Can you work these out from the model? Positions are in its coordinate system, mm. A direction names the side the tool comes from. Coordinates: 2 decimals unless noted, no trailing zeros. Write each loop counter-clockwise with the first axis right and the second up, starting at its lowest first coordinate (ties: lowest second). Pieces come first, ordered by that corner, then holes. Notation, with made-up numbers: (38.5, -39.75) -> (62.5, -39.75) arc R9 cw to (62.5, -30.75) -> close; hole circle Ø6 at (88.5, -20.5). An arc over 180 degrees is marked (long way). Use one line per item in the form item = value.
```python
from build123d import *

# Parameters (mm, degrees)
SKETCH1_R            = 1.5
SKETCH1_R_2          = 73
BOSS_EXTRUDE1_DEPTH  = 20
SKETCH7_R            = 73
SKETCH7_R_2          = 52.25
BOSS_EXTRUDE2_DEPTH  = 10
SKETCH8_R            = 73
BOSS_EXTRUDE3_DEPTH  = 10
BOSS_EXTRUDE4_DEPTH  = 20
SKETCH10_R           = 55.2
SKETCH10_R_2         = 52.25
CUT_EXTRUDE1_DEPTH   = 10
SKETCH11_R           = 40
CUT_EXTRUDE2_DEPTH   = 50
SKETCH12_R           = 3
SKETCH12_R_2         = 1.5
CUT_EXTRUDE3_DEPTH   = 3
SKETCH13_W           = 50
SKETCH13_H           = 6.823606938
BOSS_EXTRUDE5_DEPTH  = 5
BOSS_EXTRUDE6_DEPTH  = 5
BOSS_EXTRUDE7_DEPTH  = 5
BOSS_EXTRUDE8_DEPTH  = 5
SKETCH19_R           = 1.5
CUT_EXTRUDE4_DEPTH   = 5
SKETCH20_R           = 1.5
CUT_EXTRUDE5_DEPTH   = 5
SKETCH21_R           = 1.5
CUT_EXTRUDE6_DEPTH   = 5
SKETCH22_R           = 1.5
CUT_EXTRUDE7_DEPTH   = 5
SKETCH23_R           = 1.5
SKETCH23_R_2         = 1
BOSS_EXTRUDE9_DEPTH  = 5
SKETCH24_R           = 1.5
SKETCH24_R_2         = 1
BOSS_EXTRUDE10_DEPTH = 5
SKETCH25_R           = 1.5
SKETCH25_R_2         = 1
BOSS_EXTRUDE11_DEPTH = 5
SKETCH26_R           = 1.5
SKETCH26_R_2         = 1
BOSS_EXTRUDE12_DEPTH = 5


with BuildPart() as part:
    # Sketch1 → Boss-Extrude1 (new body)
    with BuildSketch(Plane(origin=(0, 0, 0), x_dir=(1, 0, 0), z_dir=(0, 1, 0))):
        with BuildLine():
            Line((77.460838348, -75.098177713), (77.460838348, 74.577424045))
            ThreePointArc((77.460838348, 74.577424045), (76.578174547, 76.708362964), (74.447235628, 77.591026765))
            Line((74.447235628, 77.591026765), (-75.22836613, 77.591026765))
            ThreePointArc((-75.22836613, 77.591026765), (-77.359305049, 76.708362964), (-78.24196885, 74.577424045))
            Line((-78.24196885, 74.577424045), (-78.24196885, -75.098177713))
            ThreePointArc((-78.24196885, -75.098177713), (-77.359305049, -77.229116632), (-75.22836613, -78.111780433))
            Line((-75.22836613, -78.111780433), (74.447235628, -78.111780433))
            ThreePointArc((74.447235628, -78.111780433), (76.578174547, -77.229116632), (77.460838348, -75.098177713))
        make_face()
        with Locations((-60.604326536, -60.47413812)):
            Circle(SKETCH1_R, mode=Mode.SUBTRACT)
        with Locations((-60.604326536, 59.953384452)):
            Circle(SKETCH1_R, mode=Mode.SUBTRACT)
        with Locations((59.823196035, 59.953384452)):
            Circle(SKETCH1_R, mode=Mode.SUBTRACT)
        with Locations((59.823196035, -60.47413812)):
            Circle(SKETCH1_R, mode=Mode.SUBTRACT)
        with Locations((-0.390565251, -0.260376834)):
            Circle(SKETCH1_R_2, mode=Mode.SUBTRACT)
    extrude(amount=BOSS_EXTRUDE1_DEPTH)

    # Sketch7 → Boss-Extrude2 (add)
    with BuildSketch(Plane(origin=(0, 20, 0), x_dir=(1, 0, 0), z_dir=(0, 1, 0))):
        with Locations((-0.390565251, -0.260376834)):
            Circle(SKETCH7_R)
        with Locations((-0.390565251, -0.260376834)):
            Circle(SKETCH7_R_2, mode=Mode.SUBTRACT)
    extrude(amount=-BOSS_EXTRUDE2_DEPTH)

    # Sketch8 → Boss-Extrude3 (add)
    with BuildSketch(Plane.XZ.offset(-10)):
        with Locations((-0.390565251, 0.260376834)):
            Circle(SKETCH8_R)
    extrude(amount=BOSS_EXTRUDE3_DEPTH)

    # Sketch9 → Boss-Extrude4 (add)
    with BuildSketch(Plane(origin=(0, 20, 0), x_dir=(1, 0, 0), z_dir=(0, 1, 0))):
        with BuildLine():
            ThreePointArc((-75.22836613, -78.111780433), (-77.359305049, -77.229116632), (-78.24196885, -75.098177713))
            Line((-78.24196885, -75.098177713), (-78.24196885, -78.111780433))
            Line((-78.24196885, -78.111780433), (-75.22836613, -78.111780433))
        make_face()
        with BuildLine():
            Line((77.460838348, -78.111780433), (77.460838348, -75.098177713))
            ThreePointArc((77.460838348, -75.098177713), (76.578174547, -77.229116632), (74.447235628, -78.111780433))
            Line((74.447235628, -78.111780433), (77.460838348, -78.111780433))
        make_face()
        with BuildLine():
            Line((77.460838348, 77.591026765), (74.447235628, 77.591026765))
            ThreePointArc((74.447235628, 77.591026765), (76.578174547, 76.708362964), (77.460838348, 74.577424045))
            Line((77.460838348, 74.577424045), (77.460838348, 77.591026765))
        make_face()
        with BuildLine():
            Line((-75.22836613, 77.591026765), (-78.24196885, 77.591026765))
            Line((-78.24196885, 77.591026765), (-78.24196885, 74.577424045))
            ThreePointArc((-78.24196885, 74.577424045), (-77.359305049, 76.708362964), (-75.22836613, 77.591026765))
        make_face()
    extrude(amount=-BOSS_EXTRUDE4_DEPTH)

    # Sketch10 → Cut-Extrude1 (cut)
    with BuildSketch(Plane(origin=(0, 20, 0), x_dir=(1, 0, 0), z_dir=(0, 1, 0))):
        with Locations((-0.390565251, -0.260376834)):
            Circle(SKETCH10_R)
        with Locations((-0.390565251, -0.260376834)):
            Circle(SKETCH10_R_2, mode=Mode.SUBTRACT)
    extrude(amount=-CUT_EXTRUDE1_DEPTH, mode=Mode.SUBTRACT)

    # Sketch11 → Cut-Extrude2 (cut)
    with BuildSketch(Plane(origin=(0, 20, 0), x_dir=(1, 0, 0), z_dir=(0, 1, 0))):
        with Locations((-0.390565251, -0.260376834)):
            Circle(SKETCH11_R)
    extrude(amount=-CUT_EXTRUDE2_DEPTH, mode=Mode.SUBTRACT)

    # Sketch12 → Cut-Extrude3 (cut)
    with BuildSketch(Plane(origin=(0, 20, 0), x_dir=(1, 0, 0), z_dir=(0, 1, 0))):
        with Locations((59.823196035, 59.953384452)):
            Circle(SKETCH12_R)
        with Locations((59.823196035, 59.953384452)):
            Circle(SKETCH12_R_2, mode=Mode.SUBTRACT)
        with Locations((-60.604326536, 59.953384452)):
            Circle(SKETCH12_R)
        with Locations((-60.604326536, 59.953384452)):
            Circle(SKETCH12_R_2, mode=Mode.SUBTRACT)
        with Locations((-60.604326536, -60.47413812)):
            Circle(SKETCH12_R)
        with Locations((-60.604326536, -60.47413812)):
            Circle(SKETCH12_R_2, mode=Mode.SUBTRACT)
        with Locations((59.823196035, -60.47413812)):
            Circle(SKETCH12_R)
        with Locations((59.823196035, -60.47413812)):
            Circle(SKETCH12_R_2, mode=Mode.SUBTRACT)
    extrude(amount=-CUT_EXTRUDE3_DEPTH, mode=Mode.SUBTRACT)

    # Sketch13 → Boss-Extrude5 (add)
    with BuildSketch(Plane.ZY.offset(78.24196885)):
        with Locations((0.260376834, 23.411803469)):
            Rectangle(SKETCH13_W, SKETCH13_H)
        Polygon((12.760376834, 32.49492606), (25.260376834, 26.823606938), (-24.739623166, 26.823606938), (-12.239623166, 32.49492606), align=None)
    extrude(amount=-BOSS_EXTRUDE5_DEPTH)

    # Sketch14 → Boss-Extrude6 (add)
    with BuildSketch(Plane(origin=(77.460838348, 0, 0), x_dir=(0, 0, -1), z_dir=(1, 0, 0))):
        Polygon((-25.260376834, 26.823606938), (-25.260376834, 20), (24.739623166, 20), (24.739623166, 26.823606938), (12.239623166, 32.49492606), (-12.760376834, 32.49492606), align=None)
    extrude(amount=-BOSS_EXTRUDE6_DEPTH)

    # Sketch17 → Boss-Extrude7 (add)
    with BuildSketch(Plane(origin=(0, 0, -77.591026765), x_dir=(-1, 0, 0), z_dir=(0, 0, -1))):
        Polygon((-77.460838348, 0), (78.24196885, 0), (78.24196885, 20), (25.390565251, 20), (25.390565251, 26.823606938), (12.890565251, 32.49492606), (-12.109434749, 32.49492606), (-24.609434749, 26.823606938), (-24.609434749, 20), (-77.460838348, 20), align=None)
    extrude(amount=-BOSS_EXTRUDE7_DEPTH)

    # Sketch18 → Boss-Extrude8 (add)
    with BuildSketch(Plane.XY.offset(78.111780433)):
        Polygon((-25.390565251, 20), (24.609434749, 20), (24.609434749, 26.823606938), (12.109434749, 32.49492606), (-12.890565251, 32.49492606), (-25.390565251, 26.823606938), align=None)
    extrude(amount=-BOSS_EXTRUDE8_DEPTH)

    # Sketch19 → Cut-Extrude4 (cut)
    with BuildSketch(Plane.ZY.offset(78.24196885)):
        with Locations((0.260376834, 26.24746303)):
            Circle(SKETCH19_R)
        with Locations((60.47413812, 10)):
            Circle(SKETCH19_R)
        with Locations((-59.953384452, 10)):
            Circle(SKETCH19_R)
    extrude(amount=-CUT_EXTRUDE4_DEPTH, mode=Mode.SUBTRACT)

    # Sketch20 → Cut-Extrude5 (cut)
    with BuildSketch(Plane(origin=(77.460838348, 0, 0), x_dir=(0, 0, -1), z_dir=(1, 0, 0))):
        with Locations((-60.47413812, 10)):
            Circle(SKETCH20_R)
        with Locations((59.953384452, 10)):
            Circle(SKETCH20_R)
        with Locations((-0.260376834, 26.24746303)):
            Circle(SKETCH20_R)
    extrude(amount=-CUT_EXTRUDE5_DEPTH, mode=Mode.SUBTRACT)

    # Sketch21 → Cut-Extrude6 (cut)
    with BuildSketch(Plane(origin=(0, 0, -77.591026765), x_dir=(-1, 0, 0), z_dir=(0, 0, -1))):
        with Locations((-59.823196035, 10)):
            Circle(SKETCH21_R)
        with Locations((0.390565251, 26.24746303)):
            Circle(SKETCH21_R)
        with Locations((60.604326536, 10)):
            Circle(SKETCH21_R)
    extrude(amount=-CUT_EXTRUDE6_DEPTH, mode=Mode.SUBTRACT)

    # Sketch22 → Cut-Extrude7 (cut)
    with BuildSketch(Plane.XY.offset(78.111780433)):
        with Locations((59.823196035, 10)):
            Circle(SKETCH22_R)
        with Locations((-0.390565251, 26.24746303)):
            Circle(SKETCH22_R)
        with Locations((-60.604326536, 10)):
            Circle(SKETCH22_R)
    extrude(amount=-CUT_EXTRUDE7_DEPTH, mode=Mode.SUBTRACT)

    # Sketch23 → Boss-Extrude9 (add)
    with BuildSketch(Plane.ZY.offset(78.24196885)):
        with Locations((60.47413812, 10)):
            Circle(SKETCH23_R)
        with Locations((60.47413812, 10)):
            Circle(SKETCH23_R_2, mode=Mode.SUBTRACT)
        with Locations((-59.953384452, 10)):
            Circle(SKETCH23_R)
        with Locations((-59.953384452, 10)):
            Circle(SKETCH23_R_2, mode=Mode.SUBTRACT)
        with Locations((0.260376834, 26.24746303)):
            Circle(SKETCH23_R)
        with Locations((0.260376834, 26.24746303)):
            Circle(SKETCH23_R_2, mode=Mode.SUBTRACT)
    extrude(amount=-BOSS_EXTRUDE9_DEPTH)

    # Sketch24 → Boss-Extrude10 (add)
    with BuildSketch(Plane.XY.offset(78.111780433)):
        with Locations((-60.604326536, 10)):
            Circle(SKETCH24_R)
        with Locations((-60.604326536, 10)):
            Circle(SKETCH24_R_2, mode=Mode.SUBTRACT)
        with Locations((-0.390565251, 26.24746303)):
            Circle(SKETCH24_R)
        with Locations((-0.390565251, 26.24746303)):
            Circle(SKETCH24_R_2, mode=Mode.SUBTRACT)
        with Locations((59.823196035, 10)):
            Circle(SKETCH24_R)
        with Locations((59.823196035, 10)):
            Circle(SKETCH24_R_2, mode=Mode.SUBTRACT)
    extrude(amount=-BOSS_EXTRUDE10_DEPTH)

    # Sketch25 → Boss-Extrude11 (add)
    with BuildSketch(Plane(origin=(77.460838348, 0, 0), x_dir=(0, 0, -1), z_dir=(1, 0, 0))):
        with Locations((-60.47413812, 10)):
            Circle(SKETCH25_R)
        with Locations((-60.47413812, 10)):
            Circle(SKETCH25_R_2, mode=Mode.SUBTRACT)
        with Locations((59.953384452, 10)):
            Circle(SKETCH25_R)
        with Locations((59.953384452, 10)):
            Circle(SKETCH25_R_2, mode=Mode.SUBTRACT)
        with Locations((-0.260376834, 26.24746303)):
            Circle(SKETCH25_R)
        with Locations((-0.260376834, 26.24746303)):
            Circle(SKETCH25_R_2, mode=Mode.SUBTRACT)
    extrude(amount=-BOSS_EXTRUDE11_DEPTH)

    # Sketch26 → Boss-Extrude12 (add)
    with BuildSketch(Plane(origin=(0, 0, -77.591026765), x_dir=(-1, 0, 0), z_dir=(0, 0, -1))):
        with Locations((-59.823196035, 10)):
            Circle(SKETCH26_R)
        with Locations((-59.823196035, 10)):
            Circle(SKETCH26_R_2, mode=Mode.SUBTRACT)
        with Locations((60.604326536, 10)):
            Circle(SKETCH26_R)
        with Locations((60.604326536, 10)):
            Circle(SKETCH26_R_2, mode=Mode.SUBTRACT)
        with Locations((0.390565251, 26.24746303)):
            Circle(SKETCH26_R)
        with Locations((0.390565251, 26.24746303)):
            Circle(SKETCH26_R_2, mode=Mode.SUBTRACT)
    extrude(amount=-BOSS_EXTRUDE12_DEPTH)


solid = part.part
```
Q1. If I drill on line 1 (Z direction, x = -59.5, y = 9); line 2 (Y direction, x = -41, z = 18.5); line 3 (X direction, y = 11, z = -23), over which ranges is the centre line in solid material (lowest first)? Write a range as from..to.
Return value:
line_1 = -77.59..-60.97, -58.94..59.46, 61.49..78.11
line_2 = 0..10
line_3 = -78.24..-50.45, 49.67..77.46
Q2. Suppose I cut it at C-C (y = 29.5). Write out the boundary of the cut face in (x, z), then the cut area to 3 significant figures.
Return value:
outline = (-78.24, -18.84) -> (-73.24, -18.84) -> (-73.24, 19.36) -> (-78.24, 19.36) -> close; (-19.49, -77.59) -> (18.71, -77.59) -> (18.71, -72.59) -> (-19.49, -72.59) -> close; (-19.49, 73.11) -> (18.71, 73.11) -> (18.71, 78.11) -> (-19.49, 78.11) -> close; (72.46, -18.84) -> (77.46, -18.84) -> (77.46, 19.36) -> (72.46, 19.36) -> close
area = 764 mm2
Q3. Thinking about a two-plate mould opening in X: for faces 1 (the flat face through (18.45, 29.62, 75.65)), 2 (the flat face through (75, 29.62, -18.58)), 3 (the flat face through (58, 17, 61)), which applies, released by +X, released by -X, zero draft, split by the parting line, or undercut?
Return value:
face_1 = released by +X
face_2 = zero draft
face_3 = undercut
Q4. For faces 4 (the flat face through (-25.391, 23, 76)), 5 (the flat face through (36.2, 10, -16.4)), 6 (the flat face through (-1, 25, 73.112)), which set-ups out of +Z, -Z, +X, -X, +Y, -Y let a thin tool reach every point of the face, with its end or its side?
Return value:
face_4 = +Z, -Z, -X, +Y
face_5 = +Y
face_6 = +X, -X, +Y
Q5. Suppose I cut it at A-A (x = 15). Write out the boundary of the cut face in (y, z), then the cut area to 3 significant figures.
Return value:
outline = (0, -77.59) -> (31.18, -77.59) -> (31.18, -72.59) -> (20, -72.59) -> (20, -52.75) -> (10, -52.75) -> (10, -36.66) -> (0, -36.66) -> close; (0, 37.18) -> (10, 37.18) -> (10, 53.27) -> (20, 53.27) -> (20, 73.11) -> (31.18, 73.11) -> (31.18, 78.11) -> (0, 78.11) -> close
area = 1,430 mm2
Q6. Will these pins go through, and if not, where does the flat tip stop? pin 1 (4 mm diameter, centred on x = 74.5, y = 23, fed in from -Z); pin 2 (1.8 mm diameter, centred on x = 60, z = 60.5, fed in from +Y); pin 3 (4 mm diameter, centred on x = -60.6, z = -59.95, fed in from +Y); pin 4 (1.6 mm diameter, centred on y = 10, z = -59.95, fed in from -X).
Return value:
pin_1 = -24.74
pin_2 = through
pin_3 = 17
pin_4 = -73.24
Q7. Suppose I cut it at D-D (y = 5). Write out the boundary of the cut face in (x, z), then the cut area to 3 significant figures.
Return value:
outline = (-78.24, -77.59) -> (77.46, -77.59) -> (77.46, 78.11) -> (-78.24, 78.11) -> close; hole circle Ø3 at (-60.6, -59.95); hole circle Ø3 at (-60.6, 60.47); hole circle Ø80 at (-0.39, 0.26); hole circle Ø3 at (59.82, -59.95); hole circle Ø3 at (59.82, 60.47)
area = 19,200 mm2
Q8. Suppose I cut it at B-B (z = 34). Write out the boundary of the cut face in (x, y), then the cut area to 3 significant figures.
Return value:
outline = (-78.24, 0) -> (-21.88, 0) -> (-21.88, 10) -> (-44.08, 10) -> (-44.08, 20) -> (-78.24, 20) -> close; (21.1, 0) -> (77.46, 0) -> (77.46, 20) -> (43.3, 20) -> (43.3, 10) -> (21.1, 10) -> close
area = 1,810 mm2
